Answer from the drawing. Dimensions are ordinates in mm from the lowest x, y and z of the part. A direction names the side the tool comes from. Round coordinates to 2 decimals unless told otherwise and drop trailing zeros. Write each loop counter-clockwise with the first axis right and the second up, starting at its lowest first coordinate (ties: lowest second). Pieces come first, ordered by that corner, then holes. Notation, with made-up numbers: M -29,19.5 L 19,19.5 A8 ccw 19,34.5 Z; hole C -27,-32.5 d3. An arc over 180 degrees is marked long. One line per item, written item: value. Start each with the question number.
(1) Section D-D (x = 36) is taken. Determine the outline of the cut face in (y, z).
(2) For a pull along Y with two mould halves and no side action, classify the marked faces 5, 6 and 7 as released by +Y, released by -Y, zero draft, split by the parting line, or undercut.
(3) Given P1, Ø6, axis at x = 13.5, y = 3, coming from the +Z side; P2, Ø6, axis at x = 3.5, z = 21, coming from the -Y side; P3, Ø1.5, axis at x = 52, y = 3.5, coming from the +Z side, each flat-ended and moving along its own axis, determine where each tip first touches the part or whether it passes through.
(4) Section C-C (x = 27.45) is taken. Determine the outline of the cut face in (y, z), plus the area to 3 significant figures.
(5) Section A-A (z = 9.5) is taken. Determine the outline of the cut face in (x, y), plus the area to 3 significant figures.
(6) Section B-B (y = 6.35) is taken. Determine the outline of the cut face in (x, z).
(7) Consider probe 1 along Y at (x, z) = (27.45, 2.05); probe 2 along X at (y, z) = (10.5, 20.5); probe 3 along Y at (x, z) = (51, 11.25). Determine where each line is inside the solid, lowest interval first.
(8) For the marked faces 1, 2, 3 and 4, determine the directions among +Z, -Z, +X, -X, +Y, -Y from which every point of the face is accessible in a straight line to the end or side of a thin tool.
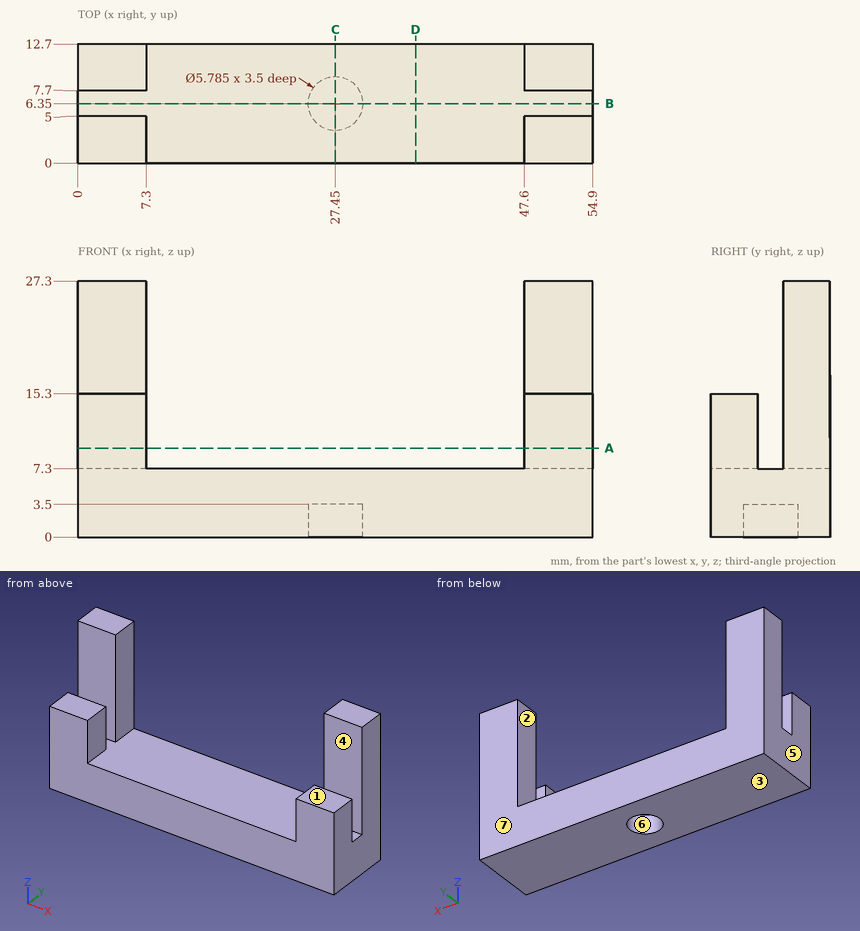
Recorded:
1. outline: M 0,0 L 12.7,0 L 12.7,7.3 L 0,7.3 Z
2. face 5: zero draft
2. face 6: undercut
2. face 7: released by +Y
3. P1: stops at z = 7.3
3. P2: stops at y = 7.7
3. P3: stops at z = 15.3
4. outline: M 0,0 L 3.46,0 L 3.46,3.5 L 9.24,3.5 L 9.24,0 L 12.7,0 L 12.7,7.3 L 0,7.3 Z
4. area: 72.5 mm2
5. outline: M 0,0 L 7.3,0 L 7.3,5 L 0,5 Z; M 0,7.7 L 7.3,7.7 L 7.3,12.7 L 0,12.7 Z; M 47.6,0 L 54.9,0 L 54.9,5 L 47.6,5 Z; M 47.6,7.7 L 54.9,7.7 L 54.9,12.7 L 47.6,12.7 Z
5. area: 146 mm2
6. outline: M 0,0 L 24.56,0 L 24.56,3.5 L 30.34,3.5 L 30.34,0 L 54.9,0 L 54.9,7.3 L 0,7.3 Z
7. probe 1: y = 0 to 3.46, 9.24 to 12.7
7. probe 2: x = 0 to 7.3, 47.6 to 54.9
7. probe 3: y = 0 to 5, 7.7 to 12.7
8. face 1: +Z, +X, -X, -Y
8. face 2: +Z, +Y, -Y
8. face 3: -Z, +X, -X, +Y, -Y
8. face 4: +Z, +X, -X
